```python
from build123d import *

# Parameters (mm, degrees)
BOSS_EXTRUDE1_DEPTH      = 114.3
BOSS_EXTRUDE1_DEPTH_BACK = 114.3
SKETCH3_R                = 12.7
SKETCH3_R_2              = 9.525


with BuildPart() as part:
    # Sketch3 → Boss-Extrude1 (new, two sides: drawn at the far end of the back side and taken through both)
    with BuildSketch(Plane.XY.offset(-BOSS_EXTRUDE1_DEPTH_BACK)):
        Circle(SKETCH3_R)
        Circle(SKETCH3_R_2, mode=Mode.SUBTRACT)
    extrude(amount=BOSS_EXTRUDE1_DEPTH + BOSS_EXTRUDE1_DEPTH_BACK)

    # SurfaceCut1
    split(bisect_by=Plane(origin=(0, -25.658113523, 104.919505636), x_dir=(1, 0, 0), z_dir=(0, -0.23755026507145888, 0.9713752475559997)), keep=Keep.BOTTOM)

    # SurfaceCut2
    split(bisect_by=Plane(origin=(0, -34.6229304, -8.467053608), x_dir=(-1, 0, 0), z_dir=(0, 0.9713752475559997, 0.23755026507145888)), keep=Keep.TOP)


solid = part.part
```
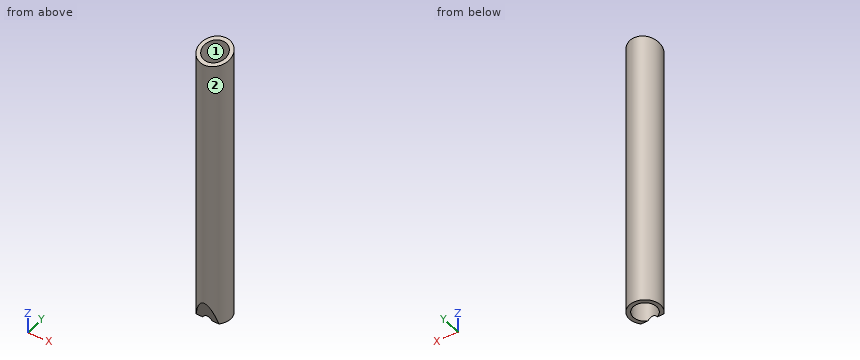
Source: CAD feature listing. Evaluate the final solid. Frame: model axes, mm. Face numbers are marked on the shaded views. Round coordinates to 2 decimals unless told otherwise and drop trailing zeros. Order: outer loops, then holes, each group sorted by start corner. A loop starts at its lowest first (then second) coordinate and runs counter-clockwise, first axis right, second up. Notation, with made-up numbers: (44, 6.25) -> (77, 6.25) arc R23 ccw to (77, 25.25) -> close; hole circle Ø1 at (-27.75, -18.75). An arc over 180 degrees is marked (long way). Use CSV: the item, a comma, the result in double quotes.
(1) Section B-B on y = 0. Return the cut outline in (x, z) (3 decimals), and give its area (3 significant figures).
Report:
outline,"(-12.7, -114.3) -> (-9.525, -114.3) -> (-9.525, 111.194) -> (-12.7, 111.194) -> close; (9.525, -114.3) -> (12.7, -114.3) -> (12.7, 111.194) -> (9.525, 111.194) -> close"
area,"1,430 mm^2"
(2) Ray query, L1, parallel to Y at x = 0, z = 3 (3 decimals); L2, parallel to Y at x = 3, z = -78.5. Return the intervals inside material, ascending.
Report:
L1,"-12.7 to -9.525, 9.525 to 12.7"
L2,"-12.34 to -9.04, 9.04 to 12.34"
(3) Pull-direction query (X, two-part tool) for the marked faces 1 and 2; classes: +X half, -X half, draft (parallel to the pull), parting line (faces both ways), or undercut.
Report:
face 1,"undercut"
face 2,"parting line"
(4) Section A-A on z = 0. Return the cut outline in (x, y) (3 decimals), and give its area (3 significant figures).
Report:
outline,"circle Ø25.4 at (0, 0); hole circle Ø19.05 at (0, 0)"
area,"222 mm^2"
(5) First-contact query: pin 1 Ø4 at (x, z) = (-5.5, 41) entering from -Y; pin 2 Ø3 at (x, z) = (-8.5, 70.5) entering from -Y; pin 3 Ø4 at (x, z) = (-6.5, -61.5) entering from +Y; pin 4 Ø15 at (x, y) = (0, 0) entering from +Z. Flat tips, straight axial feed; report the tip coordinate or a pass-through.
Report:
pin 1,"y = -12.21"
pin 2,"y = -10.6"
pin 3,"y = 11.88"
pin 4,"through"
